```python
from build123d import *

# Parameters (mm, degrees)
F0_W     = 120
F0_H     = 140
F0_W_2   = 20
F1_DEPTH = 20
F3_DEPTH = 20
F5_DEPTH = 10


# Not quite as in the source:
# - ends of sketch curves that miss each other by under 0.0002 mm in the source are joined


with BuildPart() as f1:
    # F0 (on Front) → F1 (new body)
    with BuildSketch(Plane.XZ):
        with Locations((-60, 70)):
            Rectangle(F0_W, F0_H)
        with Locations((-130, 70)):
            Rectangle(F0_W_2, F0_H)
    extrude(amount=F1_DEPTH)

    # F2 (on face) → F3 (cut)
    with BuildSketch(Plane.YZ):
        Polygon((-20, 133.6477049324), (-20, 82.2157338262), (0, 95.7159893793), (0, 120.1474493793), align=None)
        Polygon((0, 44.2840144469), (-20, 57.78427), (-20, 6.3522950676), (0, 19.8525506207), align=None)
    extrude(amount=-F3_DEPTH, mode=Mode.SUBTRACT)

    # F4 (on face) → F5 (cut)
    with BuildSketch(Plane(origin=(-140, 0, 0), x_dir=(0, -1, 0), z_dir=(-1, 0, 0))):
        with BuildLine():
            ThreePointArc((15, 75.9070515633), (10, 80.9070515633), (5, 75.9070515633))
            Line((5, 75.9070515633), (15, 75.9070515633))
        make_face()
        with BuildLine():
            Line((15, 75.9070515633), (5, 75.9070515633))
            ThreePointArc((5, 75.9070515633), (10, 70.9070515633), (15, 75.9070515633))
        make_face()
        with BuildLine():
            ThreePointArc((15, 33.7962135673), (10, 38.7962135673), (5, 33.7962135673))
            Line((5, 33.7962135673), (15, 33.7962135673))
        make_face()
        with BuildLine():
            Line((15, 33.7962135673), (5, 33.7962135673))
            ThreePointArc((5, 33.7962135673), (10, 28.7962135673), (15, 33.7962135673))
        make_face()
        with BuildLine():
            ThreePointArc((15, 118.0178895593), (10, 123.0178895593), (5, 118.0178895593))
            Line((5, 118.0178895593), (15, 118.0178895593))
        make_face()
        with BuildLine():
            Line((15, 118.0178895593), (5, 118.0178895593))
            ThreePointArc((5, 118.0178895593), (10, 113.0178895593), (15, 118.0178895593))
        make_face()
    extrude(amount=-F5_DEPTH, mode=Mode.SUBTRACT)


solid = f1.part
```
Here's how the part is built. I have some questions about the finished solid (model axes, mm). A direction names the side the tool comes from. Round coordinates to 2 decimals unless told otherwise and drop trailing zeros. Write each loop counter-clockwise with the first axis right and the second up, starting at its lowest first coordinate (ties: lowest second). Pieces come first, ordered by that corner, then holes. Notation, with made-up numbers: M -39.5,59 L -23.5,59 A32 cw -23.5,97 Z; hole C 17.25,89.25 d8. An arc over 180 degrees is marked long. Answer as CSV lines item,"result". Start each with the question number.
1. Suppose I cut it at C-C on y = -1.75. Write out the boundary of the cut face in (x, z), then the cut area to 3 significant figures.
2. Suppose I cut it at A-A on y = -10. Write out the boundary of the cut face in (x, z), then the cut area to 3 significant figures.
3. Suppose I cut it at B-B on z = 109. Write out the boundary of the cut face in (x, y).
4. I need wall thicknesses on probe 1 along Z at (x, y) = (-134, -10); probe 2 along X at (y, z) = (-11, 100); probe 3 along X at (y, z) = (-5.5, 76.5). Which ranges of each line are inside material? Lowest first, please.
5. On a 3-axis mill with a long thin cutter (end or side, diameter ignored), from which of +Z, -Z, +X, -X, +Y, -Y can I reach the whole of each face in a straight line? I mean faces 1 (the flat face through (-140, -10, 69)), 2 (the flat face through (-130, -10, 118)), 3 (the flat face through (-9.86, -10.14, 13.01)). Say none if no direction works.
6. Thinking about a two-plate mould opening in Y: for faces 4 (the cylindrical face through (-135.07, -10.65, 28.84)), 5 (the flat face through (-69, -10, 140)), 6 (the flat face through (-9.86, -9.86, 50.94)), 7 (the flat face through (-130, -10, 34)), which applies, released by +Y, released by -Y, zero draft, split by the parting line, or undercut?
7. I'm going to push flat-ended pins straight in: pin 1 Ø8 at (y, z) = (-10, 33.8) entering from +X; pin 2 Ø5 at (y, z) = (-6, 94) entering from +X; pin 3 Ø9 at (y, z) = (-10, 118.02) entering from -X. Where does each tip first touch, or does it pass through?
8. Suppose I cut it at D-D on y = -17.25. Write out the boundary of the cut face in (x, z).
Check result:
1,outline,"M -140,0 L 0,0 L 0,18.67 L -20,18.67 L -20,45.47 L 0,45.47 L 0,94.53 L -20,94.53 L -20,121.33 L 0,121.33 L 0,140 L -140,140 Z"
1,area,"18,500 mm2"
2,outline,"M -140,0 L 0,0 L 0,13.1 L -20,13.1 L -20,51.03 L 0,51.03 L 0,88.97 L -20,88.97 L -20,126.9 L 0,126.9 L 0,140 L -140,140 L -140,123.02 L -130,123.02 L -130,113.02 L -140,113.02 L -140,80.91 L -130,80.91 L -130,70.91 L -140,70.91 L -140,38.8 L -130,38.8 L -130,28.8 L -140,28.8 Z"
2,area,"17,800 mm2"
3,outline,"M -140,-20 L -20,-20 L -20,0 L -140,0 Z"
4,probe 1,"z = 0 to 28.8, 38.8 to 70.91, 80.91 to 113.02, 123.02 to 140"
4,probe 2,"x = -140 to -20"
4,probe 3,"x = -130 to 0"
5,face 1,"+Z, -Z, -X, +Y, -Y"
5,face 2,"-X"
5,face 3,"+X, -Y"
6,face 4,"undercut"
6,face 5,"zero draft"
6,face 6,"released by -Y"
6,face 7,"undercut"
7,pin 1,"stops at x = -20"
7,pin 2,"stops at x = 0"
7,pin 3,"stops at x = -130"
8,outline,"M -140,0 L 0,0 L 0,8.21 L -20,8.21 L -20,55.93 L 0,55.93 L 0,84.07 L -20,84.07 L -20,131.79 L 0,131.79 L 0,140 L -140,140 Z"
